from build123d import *

# Parameters (mm, degrees)
SKETCH_1_R      = 2.4
SKETCH_1_R_2    = 1.6
EXTRUDE_1_DEPTH = 3


with BuildPart() as part:
    # 草图1 → 凸台-拉伸1 (new body)
    with BuildSketch(Plane(origin=(0, 0, 0), x_dir=(0, 0, -1), z_dir=(1, 0, 0))):
        with BuildLine():
            Line((-52.988376737, -14.191142444), (-11.576067608, -16.887557214))
            ThreePointArc((-11.576067608, -16.887557214), (-7.935716472, -16.451026673), (-4.697384878, -14.73174665))
            Line((-4.697384878, -14.73174665), (5.632436087, -6.506846665))
            ThreePointArc((5.632436087, -6.506846665), (8.08940986, 2.62041481), (0.591065641, 8.375278503))
            Line((0.591065641, 8.375278503), (-51.299056641, 11.753918697))
            Line((-51.299056641, 11.753918697), (-52.988376737, -14.191142444))
        make_face()
        with Locations((0.038787918, -0.106760716)):
            Circle(SKETCH_1_R, mode=Mode.SUBTRACT)
        with Locations((-47.567404172, 7.502475429)):
            Circle(SKETCH_1_R_2, mode=Mode.SUBTRACT)
        with Locations((-20.796098395, -12.278757773)):
            Circle(SKETCH_1_R_2, mode=Mode.SUBTRACT)
        with Locations((-23.618116965, 5.943103032)):
            Circle(SKETCH_1_R_2, mode=Mode.SUBTRACT)
        with Locations((-48.73693347, -10.459489976)):
            Circle(SKETCH_1_R_2, mode=Mode.SUBTRACT)
    extrude(amount=EXTRUDE_1_DEPTH)


solid = part.part
For this review, take the finished solid that the model builds, in its own axes (mm). Give positions to 0.01 mm unless a question says otherwise; leave off trailing zeros. Loops run counter-clockwise (first coordinate to the right, second up) from the corner with the lowest first, then second, coordinate; pieces in that order, holes last.
Item 1: Take a section at B-B, the plane x = 1.25. State the section outline as (y, z) points, and give its area (3 significant figures).
Item 2: Take a section at D-D, the plane y = -5.75. State the section outline as (x, z) points.
Item 3: For line 1 along Z through (x, y) = (2.4, 1.75); line 2 along Y through (x, z) = (1.95, 1); line 3 along Z through (x, y) = (1.9, -11.75), list the stretches that pass through material, from the lowest coordinate up.
Item 4: Take a section at A-A, the plane y = -1.25. State the section outline as (x, z) points, and give its area (3 significant figures).
Item 5: Insertion check: pin 1 (1.5 mm diameter, centred on x = 2, y = -11.5, fed in from +Z); pin 2 (2.5 mm diameter, centred on y = -10.46, z = 48.74, fed in from +X). Each pin has a flat end and moves straight along its axis. Give the tip position at first contact, or say it passes through.
Item 6: Take a section at C-C, the plane z = 24. State the section outline as (x, y) points.
Item 7: Draft analysis for pull direction Y (two halves, no side actions). For faces 1 (the cylindrical face through (1.479, -10.389, 50.335)), 2 (the flat face through (0, -2, 23)), 3 (the cylindrical face through (1.479, -16.466, 7.985)), state which applies: +Y half, -Y half, draft (parallel to the pull), parting line (faces both ways), or undercut.
Calculated:
1. outline: (-16.89, 11.58) arc R10 ccw to (-14.73, 4.7) - (-6.51, -5.63) arc R8.5 ccw to (8.38, -0.59) - (11.75, 51.3) - (-14.19, 52.99) - close; hole circle Ø3.2 at (-12.28, 20.8); hole circle Ø3.2 at (-10.46, 48.74); hole circle Ø4.8 at (-0.11, -0.04); hole circle Ø3.2 at (5.94, 23.62); hole circle Ø3.2 at (7.5, 47.57)
1. area: 1,400 mm2
2. outline: (0, -6.4) - (3, -6.4) - (3, 52.44) - (0, 52.44) - close
3. line 1: z = -8.33 to -1.56, 1.48 to 51.95
3. line 2: y = -11.79 to -2.27, 2.06 to 8.48
3. line 3: z = 0.95 to 19.29, 22.31 to 47.79, 49.68 to 52.83
4. outline: (0, -8.46) - (3, -8.46) - (3, -2.15) - (0, -2.15) - close; (0, 2.07) - (3, 2.07) - (3, 52.15) - (0, 52.15) - close
4. area: 169 mm2
5. pin 1: stops at z = 52.86
5. pin 2: passes through
6. outline: (0, -16.08) - (3, -16.08) - (3, 4.39) - (0, 4.39) - close; (0, 7.5) - (3, 7.5) - (3, 9.98) - (0, 9.98) - close
7. face 1: undercut
7. face 2: draft
7. face 3: -Y half
